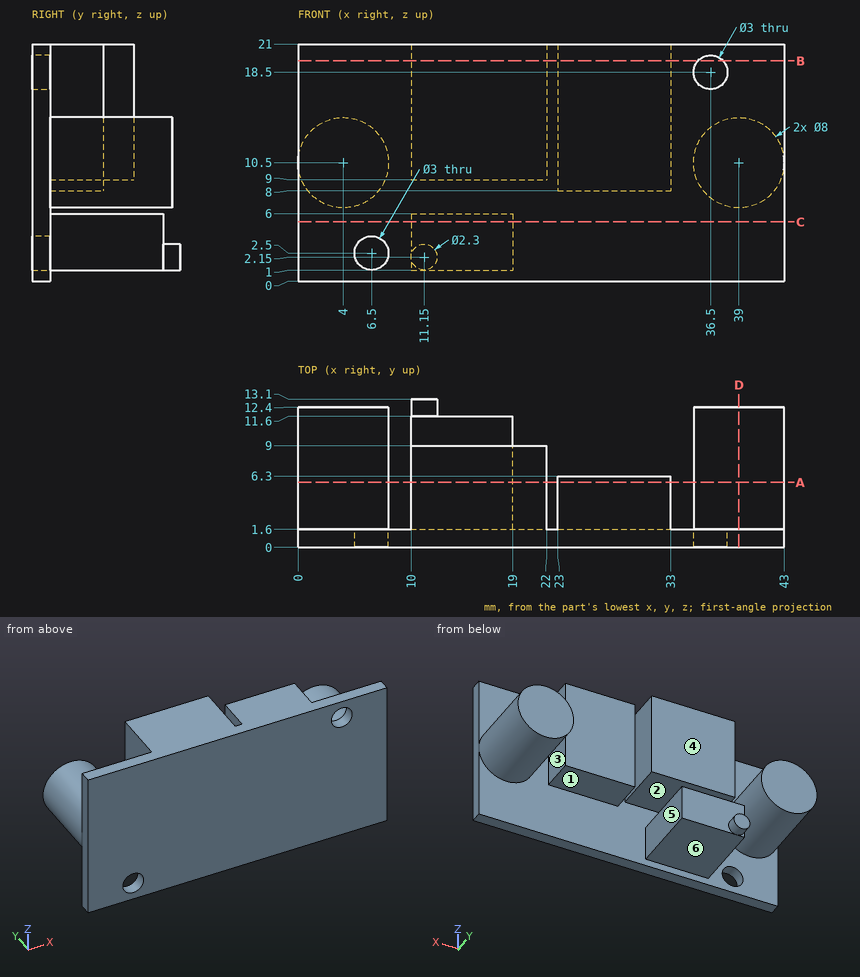
For this review, use the dimensioned drawing (mm, ordinates from the lowest corner) and the shaded views. A direction names the side the tool comes from. Give positions to 0.01 mm unless a question says otherwise; leave off trailing zeros. Loops run counter-clockwise (first coordinate to the right, second up) from the corner with the lowest first, then second, coordinate; pieces in that order, holes last.
Item 1: Draft analysis for pull direction X (two halves, no side actions). For the marked faces 4, 5 and 6, state which applies: +X half, -X half, draft (parallel to the pull), parting line (faces both ways), or undercut.
Item 2: Insertion check: pin 1 (6.5 mm diameter, centred on x = 6, z = 8.5, fed in from +Y); pin 2 (2 mm diameter, centred on y = 8, z = 9.5, fed in from -X); pin 3 (2 mm diameter, centred on y = 3.5, z = 17, fed in from +X); pin 4 (3.5 mm diameter, centred on x = 15.5, y = 6, fed in from -Z). Each pin has a flat end and moves straight along its axis. Give the tip position at first contact, or say it passes through.
Item 3: Tool access review of the marked faces 1, 2 and 3: name each direction out of +Z, -Z, +X, -X, +Y, -Y from which nothing blocks a thin tool from reaching the whole face with its end or side.
Item 4: Take a section at C-C, the plane z = 5.25. State the section outline as (x, y) points, and give its area (3 significant figures).
Item 5: Take a section at B-B, the plane z = 19.5. State the section outline as (x, y) points, and give its area (3 significant figures).
Item 6: Take a section at A-A, the plane y = 5.75. State the section outline as (x, z) points.
Item 7: Take a section at D-D, the plane x = 39. State the section outline as (y, z) points.
Item 8: For line 1 along X through (y, z) = (0.9, 2.5); line 2 along X through (y, z) = (3.75, 20); line 3 along X through (y, z) = (6, 9.5), list the stretches that pass through material, from the lowest coordinate up.
Calculated:
1. face 4: undercut
1. face 5: +X half
1. face 6: draft
2. pin 1: stops at y = 12.4
2. pin 2: stops at x = 0
2. pin 3: stops at x = 33
2. pin 4: stops at z = 1
3. face 1: -Z, +Y
3. face 2: +Y
3. face 3: +Z, -Z, +Y
4. outline: (0, 0) - (43, 0) - (43, 1.6) - (19, 1.6) - (19, 11.6) - (10, 11.6) - (10, 1.6) - (0, 1.6) - close
4. area: 159 mm2
5. outline: (0, 0) - (35.38, 0) - (35.38, 1.6) - (33, 1.6) - (33, 6.3) - (23, 6.3) - (23, 1.6) - (22, 1.6) - (22, 9) - (10, 9) - (10, 1.6) - (0, 1.6) - close; (37.62, 0) - (43, 0) - (43, 1.6) - (37.62, 1.6) - close
5. area: 201 mm2
6. outline: circle Ø8 at (4, 10.5); (10, 1) - (19, 1) - (19, 6) - (10, 6) - close; (10, 9) - (22, 9) - (22, 21) - (10, 21) - close; (23, 8) - (33, 8) - (33, 21) - (23, 21) - close; circle Ø8 at (39, 10.5)
7. outline: (0, 0) - (1.6, 0) - (1.6, 6.5) - (12.4, 6.5) - (12.4, 14.5) - (1.6, 14.5) - (1.6, 21) - (0, 21) - close
8. line 1: x = 0 to 5, 8 to 43
8. line 2: x = 10 to 22, 23 to 33
8. line 3: x = 0.13 to 7.87, 10 to 22, 23 to 33, 35.13 to 42.87
